Autodesk Inventor part; units mm, degrees
ref_plane "YZ Plane" through (0, 0, 0) normal (1, 0, 0) x (0, 1, 0)
ref_plane "XZ Plane" through (0, 0, 0) normal (0, 1, 0) x (-1, 0, 0)
ref_plane "XY Plane" through (0, 0, 0) normal (0, 0, 1) x (1, 0, 0)
sketch "Sketch1" plane through (0, 0, 0) normal (1, 0, 0) x (0, 1, 0)
  line L0 (0, 0) -> (57.15, 0)
  line L1 (57.15, 0) -> (57.15, 193.675)
  line L2 (57.15, 193.675) -> (0, 193.675)
  line L3 (0, 193.675) -> (0, 0)
  dimension "d0" = 57.15
  dimension "d1" = 193.675
extrude "Extrusion1" add sketch "Sketch1" along normal blind 173.0375
sketch "Sketch3" plane through (0, 0, 0) normal (0, 0, -1) x (-1, 0, 0)
  line L0 (-173.0375, 57.15) -> (-173.0375, 0)
  line L1 (-173.0375, 44.45) -> (-128.5875, 0)
  line L2 (-173.0375, 44.45) -> (-110.1757, 44.45) construction
  line L3 (-128.5875, 0) -> (-173.0375, 0)
  line L4 (-173.0375, 0) -> (-173.0375, 44.45)
  point P0 (0, 0)
  dimension "d9" = 45
  dimension "d10" = 12.7
  dimension "d11" = 44.45
extrude "Extrusion3" cut sketch "Sketch3" against normal up to surface (193.675 mm away)
properties part number "3-80" material "Granite, Cut, Polished"
The listing builds one solid part. Answer for the finished solid, in the listing's coordinates (mm). Coordinates: 2 decimals unless noted, no trailing zeros. Order: outer loops, then holes, each group sorted by start corner. A loop starts at its lowest first (then second) coordinate and runs counter-clockwise, first axis right, second up.
Q1. A cutting plane is placed at A-A, the plane z = 143. Write down the section's boundary in (x, y).
Q2. Consider line 1 (X direction, y = 24.5, z = 165); line 2 (X direction, y = 4, z = 63); line 3 (Y direction, x = 140, z = 157). Determine where each line is inside the solid, lowest interval first.
Q3. A cutting plane is placed at B-B, the plane y = 27. Write down the section's boundary in (x, z) (1 decimal), and give its area (3 significant figures).
Q4. Given P1, Ø1, axis at y = 39.5, z = 149.5, coming from the -X side; P2, Ø12, axis at y = 25, z = 20, coming from the +X side, each flat-ended and moving along its own axis, determine where each tip first touches the part or whether it passes through.
Answers follow:
1. outline: (0, 0) - (128.59, 0) - (173.04, 44.45) - (173.04, 57.15) - (0, 57.15) - close
2. line 1: x = 0 to 153.09
2. line 2: x = 0 to 132.59
2. line 3: y = 11.41 to 57.15
3. outline: (0, 0) - (155.6, 0) - (155.6, 193.7) - (0, 193.7) - close
3. area: 30,100 mm2
4. P1: stops at x = 0
4. P2: stops at x = 159.59
